The listing builds one solid part. Answer for the finished solid, in the listing's coordinates (mm). Face numbers are marked on the shaded views. A direction names the side the tool comes from. Coordinates: 2 decimals unless noted, no trailing zeros. Order: outer loops, then holes, each group sorted by start corner. A loop starts at its lowest first (then second) coordinate and runs counter-clockwise, first axis right, second up. Notation, with made-up numbers: (28.25, 86.5) - (73.25, 86.5) arc R27 cw to (73.25, 120.5) - close; hole circle Ø11 at (26.25, -32.5). An arc over 180 degrees is marked (long way). Use a Markdown table: item, result. Add a question column.
Item 1: Find the intervals of material crossed by line 1 along Z through (x, y) = (-18, -23); line 2 along X through (y, z) = (-44.5, 5); line 3 along Y through (x, z) = (4.5, 4.5), in increasing order.
Item 2: The part is cut by section A-A, the plane y = -20.5. Give the vertices of the cut face in (x, z), then the cut area to 3 significant figures.
Item 3: The part is cut by section D-D, the plane x = -14. Give the vertices of the cut face in (y, z), then the cut area to 3 significant figures.
Item 4: The part is cut by section B-B, the plane z = 36.5. Give the vertices of the cut face in (x, y), then the cut area to 3 significant figures.
Item 5: The part is cut by section C-C, the plane x = 4. Give the vertices of the cut face in (y, z), then the cut area to 3 significant figures.
Item 6: For the marked faces 1 and 2, determine the directions among +Z, -Z, +X, -X, +Y, -Y from which every point of the face is accessible in a straight line to the end or side of a thin tool.
Item 7: Flat-ended cylindrical pins translate along their axes: P1, Ø1, axis at x = 0.5, y = -18, coming from the +Z side; P2, Ø12, axis at x = -3, z = 41, coming from the -Y side. Find the tip coordinate at first contact, or state that the pin passes through.
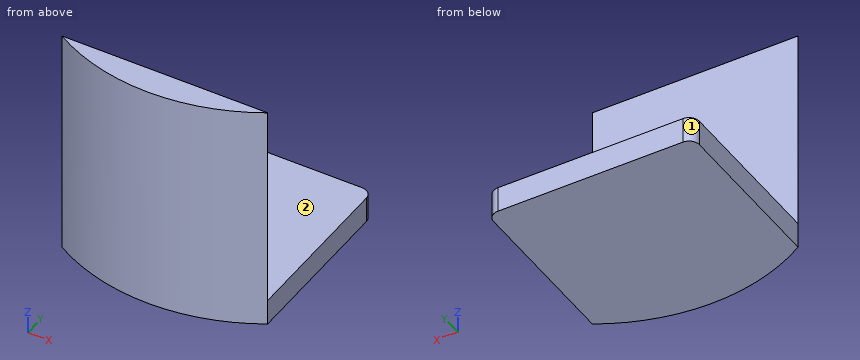
from build123d import *

# Parameters (mm, degrees)
BOSS_EXTRUDE1_DEPTH = 57.15
SKETCH2_W           = 50.8
SKETCH2_H           = 6.35
BOSS_EXTRUDE2_DEPTH = 43.18
FILLET1_R           = 2.54


with BuildPart() as part:
    # Sketch1 → Boss-Extrude1 (new body)
    with BuildSketch(Plane.XY):
        with BuildLine():
            Line((-25.4, -42.521299369), (25.4, -42.521299369))
            ThreePointArc((25.4, -42.521299369), (0, -49.53), (-25.4, -42.521299369))
        make_face()
    extrude(amount=BOSS_EXTRUDE1_DEPTH)

    # Sketch2 → Boss-Extrude2 (add)
    with BuildSketch(Plane(origin=(0, -42.521299369, 0), x_dir=(1, 0, 0), z_dir=(0, 1, 0))):
        with Locations((0, -3.175)):
            Rectangle(SKETCH2_W, SKETCH2_H)
    extrude(amount=BOSS_EXTRUDE2_DEPTH)

    # Fillet1
    fillet1_edges = [part.edges().sort_by_distance(p)[0] for p in [
        (-25.4, 0.658700631, 3.175),
        (25.4, 0.658700631, 3.175),
    ]]
    fillet(fillet1_edges, radius=FILLET1_R)


solid = part.part
Solution:
| question | item | result |
|---|---|---|
| 1 | line 1 | z = 0 to 6.35 |
| 1 | line 2 | x = -21.75 to 21.75 |
| 1 | line 3 | y = -49.33 to 0.66 |
| 2 | outline | (-25.4, 0) - (25.4, 0) - (25.4, 6.35) - (-25.4, 6.35) - close |
| 2 | area | 323 mm2 |
| 3 | outline | (-47.51, 0) - (0.66, 0) - (0.66, 6.35) - (-42.52, 6.35) - (-42.52, 57.15) - (-47.51, 57.15) - close |
| 3 | area | 559 mm2 |
| 4 | outline | (-25.4, -42.52) arc R49.53 ccw to (25.4, -42.52) - close |
| 4 | area | 241 mm2 |
| 5 | outline | (-49.37, 0) - (0.66, 0) - (0.66, 6.35) - (-42.52, 6.35) - (-42.52, 57.15) - (-49.37, 57.15) - close |
| 5 | area | 665 mm2 |
| 6 | face 1 | +Z, -Z, -X, +Y |
| 6 | face 2 | +Z, +X, -X, +Y |
| 7 | P1 | stops at z = 6.35 |
| 7 | P2 | stops at y = -49.53 |
